Design review of the part built by this model. Coordinates are the model's own, in mm. A direction names the side the tool comes from. Coordinates: 2 decimals unless noted, no trailing zeros. Order: outer loops, then holes, each group sorted by start corner. A loop starts at its lowest first (then second) coordinate and runs counter-clockwise, first axis right, second up. Notation, with made-up numbers: (29.25, 16.25) -> (81.25, 16.25) arc R21 ccw to (81.25, 32.25) -> close; hole circle Ø10 at (42, 16). An arc over 180 degrees is marked (long way). Write item = value, one per line.
```python
from build123d import *

# Parameters (mm, degrees)
SKETCH2_W      = 0.625748312
SKETCH2_H      = 0.221900722
REVOLVE5_ANGLE = 180


with BuildPart() as part:
    # Sketch1 → Revolve4 (revolve)
    with BuildSketch(Plane.XY, mode=Mode.PRIVATE) as revolve4_sk:
        Polygon((-12.065, 11.43), (-12.065, 10.16), (-1.079269363, 9.259170088), (-1.079269363, 0), (0.635, 0), (0.635, 9.1186), (11.979982671, 8.188311421), (11.979982671, 7.399559782), (17.704559016, 7.399559782), (17.704559016, 8.0772), (13.335, 8.0772), (13.335, 9.3472), align=None)
    revolve(revolve4_sk.sketch.rotate(Axis((44.726440805, 0, 0), (-1, 0, 0)), 90), axis=Axis((44.726440805, 0, 0), (-1, 0, 0)))

    # Sketch2 → Revolve5 (revolve)
    with BuildSketch(Plane(origin=(0.635, 0, 0), x_dir=(0, 0, -1), z_dir=(1, 0, 0))):
        with Locations((0, 0.897225516)):
            Rectangle(SKETCH2_W, SKETCH2_H)
    revolve(axis=Axis((0.635, 0, 0.312874156), (0, 0, -1)), revolution_arc=REVOLVE5_ANGLE)


solid = part.part
```
(1) The part is to be moulded in two halves that separate along Z. For faces 4 (the flat face through (13.335, 3, -8)), 5 (the cylindrical face through (15.489, -2.426, -7.704)), 6 (the flat face through (-1.079, 0, 0)), say which applies: released by +Z, released by -Z, zero draft, split by the parting line, or undercut.
Report:
face_4 = zero draft
face_5 = split by the parting line
face_6 = undercut
(2) For faces 1 (the cylindrical face through (1.643, 0.022, -0.004)), 2 (the flat face through (11.98, 6.6, 3.7)), 3 (the conical face through (-5.275, 9.375, 2.082)), list the 3-axis set-ups (+Z, -Z, +X, -X, +Y, -Y) from which the entire face can be reached by the end or side of a thin tool; tool diameter is ignored.
Report:
face_1 = +X
face_2 = none
face_3 = -X
(3) We need section C-C (x = -6.75). Write out the cut boundary in (y, z), and give its area (3 significant figures).
Report:
outline = circle Ø21.99 at (0, 0); hole circle Ø19.45 at (0, 0)
area = 82.7 mm²
(4) Insertion check: pin 1 (1 mm diameter, centred on x = 7, z = 1, fed in from +Y); pin 2 (10 mm diameter, centred on x = -8.5, z = -9, fed in from -Y); pin 3 (8 mm diameter, centred on x = 12.5, z = 3, fed in from +Y). Each pin has a flat end and moves straight along its axis. Give the tip position at first contact, or say it passes through.
Report:
pin_1 = 9.87
pin_2 = -10.44
pin_3 = 9.66
(5) For L1, parallel to Y at x = 14.85, z = 0; L2, parallel to X at y = -5, z = 6 (3 decimals); L3, parallel to Z at x = -7.5, y = -8, list the stretches that pass through material, from the lowest coordinate up.
Report:
L1 = -8.08 to -7.4, 7.4 to 8.08
L2 = -1.079 to 0.635, 11.98 to 17.705
L3 = -7.63 to -5.64, 5.64 to 7.63
(6) We need section A-A (y = 0). Write out the cut boundary in (x, z) (3 decimals), and give its area (3 significant figures).
Report:
outline = (-12.065, -11.43) -> (13.335, -9.347) -> (13.335, -8.077) -> (17.705, -8.077) -> (17.705, -7.4) -> (11.98, -7.4) -> (11.98, -8.188) -> (0.635, -9.119) -> (0.635, 9.119) -> (11.98, 8.188) -> (11.98, 7.4) -> (17.705, 7.4) -> (17.705, 8.077) -> (13.335, 8.077) -> (13.335, 9.347) -> (-12.065, 11.43) -> (-12.065, 10.16) -> (-1.079, 9.259) -> (-1.079, -9.259) -> (-12.065, -10.16) -> close; (1.421, -0.313) -> (1.643, -0.313) -> (1.643, 0.313) -> (1.421, 0.313) -> close
area = 104 mm²
(7) We need section B-B (x = 14.25). Write out the cut boundary in (y, z).
Report:
outline = circle Ø16.15 at (0, 0); hole circle Ø14.8 at (0, 0)
